Input: dimensioned drawing with shaded views. Units: mm. Origin: part minimum x, y, z. A direction names the side the tool comes from. Coordinates: 2 decimals unless noted, no trailing zeros. Loops run counter-clockwise (first coordinate to the right, second up) from the corner with the lowest first, then second, coordinate; pieces in that order, holes last.
Item 1: Section query D-D, the plane x = 6.25. Return the cut outline in (y, z), then the cut area to 3 significant figures.
Item 2: Section query C-C, the plane z = 3.5. Return the cut outline in (x, y).
Item 3: Reachability of the marked faces 1 and 2 from +Z, -Z, +X, -X, +Y, -Y: full face, straight path, thin tool, end or side. Return the list, or none.
Item 4: Pin query (flat end, axial travel): pin 1 Ø3 at (x, z) = (4, 22) entering from +Y (3 decimals); pin 2 Ø1.5 at (y, z) = (18, 23.5) entering from -X; pin 3 Ø6 at (y, z) = (11.5, 33) entering from +X. Return the tip coordinate at first contact, or that it passes through.
Item 5: Section query A-A, the plane y = 10.5. Return the cut outline in (x, z), then the cut area to 3 significant figures.
Item 6: Line query: probe 1 along Y at (x, z) = (10.5, 35.5); probe 2 along Z at (x, y) = (9.75, 19); probe 3 along X at (y, z) = (3.25, 11). Output: solid intervals per line, ascending.
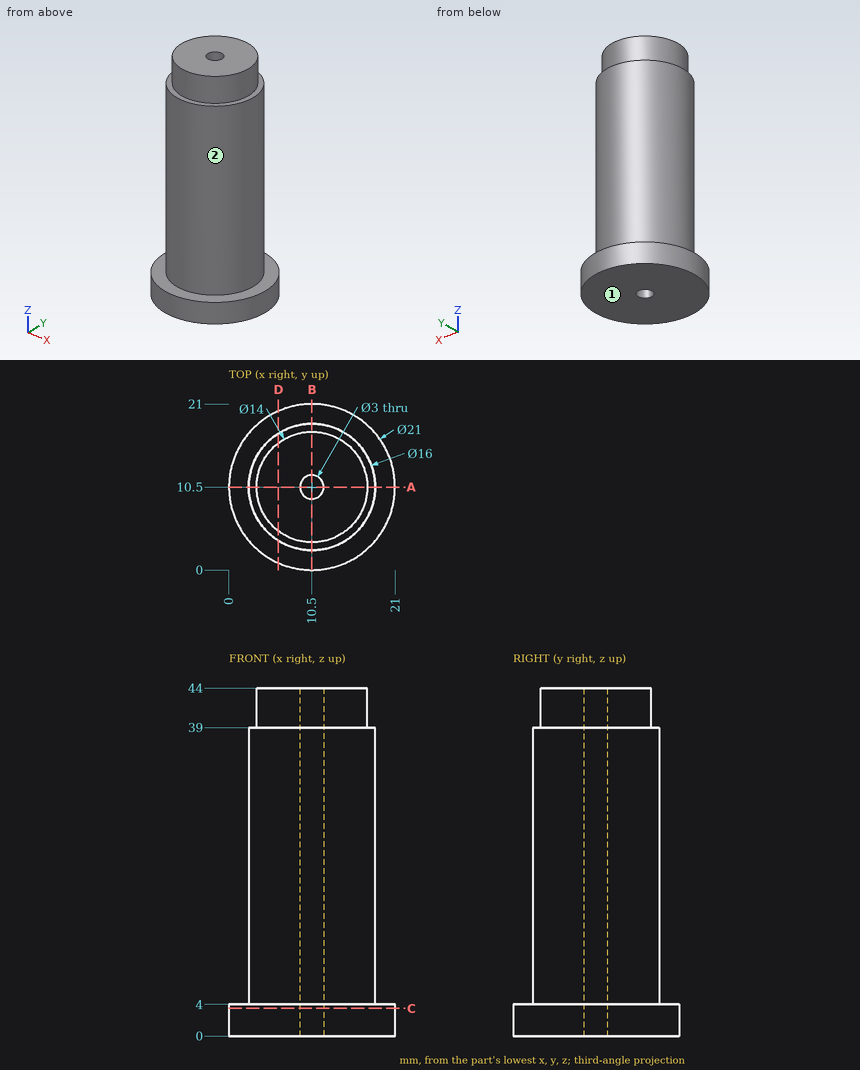
Verdict:
1. outline: (0.9, 0) - (20.1, 0) - (20.1, 4) - (17.28, 4) - (17.28, 39) - (16.06, 39) - (16.06, 44) - (4.94, 44) - (4.94, 39) - (3.72, 39) - (3.72, 4) - (0.9, 4) - close
1. area: 607 mm2
2. outline: circle Ø21 at (10.5, 10.5); hole circle Ø3 at (10.5, 10.5)
3. face 1: -Z, +X, -X, +Y, -Y
3. face 2: +Z
4. pin 1: stops at y = 16.745
4. pin 2: stops at x = 6.21
4. pin 3: stops at x = 18.5
5. outline: (0, 0) - (9, 0) - (9, 44) - (3.5, 44) - (3.5, 39) - (2.5, 39) - (2.5, 4) - (0, 4) - close; (12, 0) - (21, 0) - (21, 4) - (18.5, 4) - (18.5, 39) - (17.5, 39) - (17.5, 44) - (12, 44) - close
5. area: 582 mm2
6. probe 1: y = 2.5 to 9, 12 to 18.5
6. probe 2: z = 0 to 4
6. probe 3: x = 7.12 to 13.88
